The listing builds one solid part. Answer for the finished solid, in the listing's coordinates (mm). Round coordinates to 2 decimals unless told otherwise and drop trailing zeros. Write each loop counter-clockwise with the first axis right and the second up, starting at its lowest first coordinate (ties: lowest second). Pieces come first, ordered by that corner, then holes. Notation, with made-up numbers: M 51,35.5 L 83,35.5 A26 ccw 83,65.5 Z; hole C -28,41.25 d8. An arc over 180 degrees is marked long. One line per item, written item: value. Start each with the question number.
(1) Consider probe 1 along Z at (x, y) = (9, 0) (3 decimals); probe 2 along Z at (x, y) = (120, 0) (3 decimals); probe 3 along X at (y, z) = (-2.5, 0.5). Determine where each line is inside the solid, lowest interval first.
(2) Section A-A (x = 46) is taken. Determine the outline of the cut face in (y, z) (3 decimals).
(3) Given P1, Ø3, axis at x = 58.5, y = -2.5, coming from the +Z side; P2, Ø2, axis at y = 0, z = 0, coming from the -X side; P3, Ø3.5, axis at y = 0.5, z = 2, coming from the -X side, each flat-ended and moving along its own axis, determine where each tip first touches the part or whether it passes through.
(4) Section B-B (x = 83) is taken. Determine the outline of the cut face in (y, z) (3 decimals), plus the area to 3 significant figures.
```python
from build123d import *

# Parameters (mm, degrees)
F0_R     = 3.175
F1_DEPTH = 127
F3_D     = 2.5781
F3_DEPTH = 12.7
F3_TIP   = 0.774539381
F5_DEPTH = 76.2


with BuildPart() as f1:
    # F0 (on Right) → F1 (new body)
    with BuildSketch(Plane.YZ):
        Circle(F0_R)
    extrude(amount=F1_DEPTH)

    # F3
    with Locations(Plane.YZ.offset(127)):
        with Locations((0, 0)):
            Hole(F3_D / 2, depth=F3_DEPTH)
            with Locations((0, 0, -(F3_DEPTH + F3_TIP / 2))):  # 118° drill point
                Cone(0, F3_D / 2, F3_TIP, mode=Mode.SUBTRACT)

    # F4 (on face) → F5 (cut)
    with BuildSketch(Plane(origin=(0, 0, 0), x_dir=(0, -1, 0), z_dir=(-1, 0, 0))):
        with BuildLine():
            ThreePointArc((-0.8255, 0), (0, 0.8255), (0.8255, 0))
            Line((0.8255, 0), (3.175, 0))
            ThreePointArc((3.175, 0), (0, 3.175), (-3.175, 0))
            Line((-3.175, 0), (-0.8255, 0))
        make_face()
        with BuildLine():
            Line((-0.8255, 0), (0.8255, 0))
            ThreePointArc((0.8255, 0), (0, 0.8255), (-0.8255, 0))
        make_face()
    extrude(amount=-F5_DEPTH, mode=Mode.SUBTRACT)


solid = f1.part
```
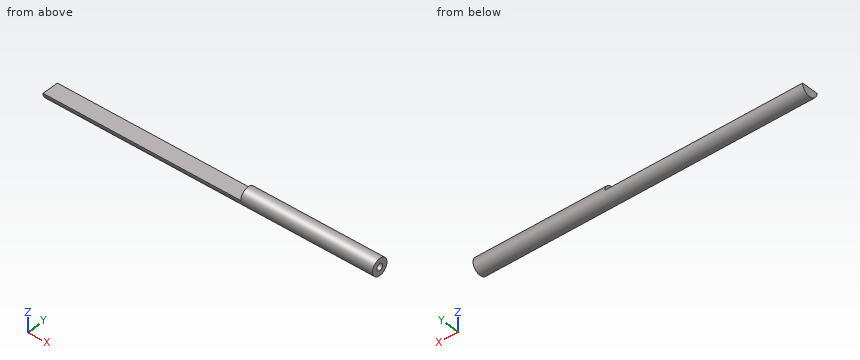
Recorded:
1. probe 1: z = -3.175 to 0
1. probe 2: z = -3.175 to -1.289, 1.289 to 3.175
1. probe 3: x = 76.2 to 127
2. outline: M -3.175,0 A3.175 ccw 3.175,0 Z
3. P1: stops at z = 0
3. P2: stops at x = 0
3. P3: stops at x = 76.2
4. outline: C 0,0 d6.35
4. area: 31.7 mm2
